from build123d import *

# Parameters (mm, degrees)
BOSS_EXTRUDE1_DEPTH = 400
SKETCH3_W           = 100
SKETCH3_H           = 300
CUT_EXTRUDE1_DEPTH  = 400
SKETCH4_W           = 60
SKETCH4_H           = 340
CUT_EXTRUDE2_DEPTH  = 400
SKETCH5_W           = 70
SKETCH5_H           = 340
CUT_EXTRUDE4_DEPTH  = 118
SKETCH6_R           = 5
CUT_EXTRUDE5_DEPTH  = 543
SKETCH7_R           = 5
CUT_EXTRUDE6_DEPTH  = 193
SKETCH8_R           = 10
CUT_EXTRUDE7_DEPTH  = 20
SKETCH9_W           = 100
SKETCH9_H           = 180
BOSS_EXTRUDE2_DEPTH = 20
SKETCH11_R          = 1
CUT_EXTRUDE8_DEPTH  = 26.5
SKETCH12_R          = 3.5
CUT_EXTRUDE9_DEPTH  = 35


with BuildPart() as part:
    # Sketch2 → Boss-Extrude1 (new body)
    with BuildSketch(Plane(origin=(0, 0, 0), x_dir=(1, 0, 0), z_dir=(0, 1, 0))):
        Polygon((0, 0), (0, 100), (20, 100), (20, 20), (180, 20), (180, 150), (200, 150), (200, 0), align=None)
    extrude(amount=-BOSS_EXTRUDE1_DEPTH)

    # Sketch3 → Cut-Extrude1 (cut)
    with BuildSketch(Plane.XY):
        with Locations((100, -200)):
            Rectangle(SKETCH3_W, SKETCH3_H)
    extrude(amount=-CUT_EXTRUDE1_DEPTH, mode=Mode.SUBTRACT)

    # Sketch4 → Cut-Extrude2 (cut)
    with BuildSketch(Plane.ZY):
        with Locations((-50, -200)):
            Rectangle(SKETCH4_W, SKETCH4_H)
    extrude(amount=-CUT_EXTRUDE2_DEPTH, mode=Mode.SUBTRACT)

    # Sketch5 → Cut-Extrude4 (cut)
    with BuildSketch(Plane(origin=(200, 0, 0), x_dir=(0, 0, -1), z_dir=(1, 0, 0))):
        with Locations((115, -200)):
            Rectangle(SKETCH5_W, SKETCH5_H)
    extrude(amount=-CUT_EXTRUDE4_DEPTH, mode=Mode.SUBTRACT)

    # Sketch6 → Cut-Extrude5 (cut)
    with BuildSketch(Plane(origin=(0, 0, 0), x_dir=(1, 0, 0), z_dir=(0, 1, 0))):
        with Locations(Location((190, 142, 0), (0, 0, 90))):
            Circle(SKETCH6_R)
        with Locations(Location((190, 129, 0), (0, 0, 90))):
            Circle(SKETCH6_R)
        with Locations(Location((190, 116, 0), (0, 0, 90))):
            Circle(SKETCH6_R)
        with Locations(Location((190, 103, 0), (0, 0, 90))):
            Circle(SKETCH6_R)
        with Locations(Location((190, 90, 0), (0, 0, 90))):
            Circle(SKETCH6_R)
    extrude(amount=-CUT_EXTRUDE5_DEPTH, mode=Mode.SUBTRACT)

    # Sketch7 → Cut-Extrude6 (cut)
    with BuildSketch(Plane.ZY):
        with Locations((-90, -80)):
            Circle(SKETCH7_R)
        with Locations((-90, -320)):
            Circle(SKETCH7_R)
    extrude(amount=-CUT_EXTRUDE6_DEPTH, mode=Mode.SUBTRACT)

    # Sketch8 → Cut-Extrude7 (cut)
    with BuildSketch(Plane.XY):
        with Locations((180, -60)):
            Circle(SKETCH8_R)
        with Locations((20, -60)):
            Circle(SKETCH8_R)
        with Locations((180, -340)):
            Circle(SKETCH8_R)
        with Locations((20, -340)):
            Circle(SKETCH8_R)
    extrude(amount=-CUT_EXTRUDE7_DEPTH, mode=Mode.SUBTRACT)

    # Sketch9 → Boss-Extrude2 (add)
    with BuildSketch(Plane.XY):
        with Locations((100, -200)):
            Rectangle(SKETCH9_W, SKETCH9_H)
    extrude(amount=-BOSS_EXTRUDE2_DEPTH)

    # Sketch11 → Cut-Extrude8 (cut, symmetric)
    with BuildSketch(Plane.XY):
        with Locations((75, -220)):
            Circle(SKETCH11_R)
        with Locations((123.17, -220)):
            Circle(SKETCH11_R)
    extrude(amount=CUT_EXTRUDE8_DEPTH, both=True, mode=Mode.SUBTRACT)

    # Sketch12 → Cut-Extrude9 (cut)
    with BuildSketch(Plane.XY):
        with Locations((190, -185)):
            Circle(SKETCH12_R)
    cut_extrude9 = extrude(amount=-CUT_EXTRUDE9_DEPTH, mode=Mode.SUBTRACT)

    # Mirror1: Cut-Extrude9 across plane
    add(cut_extrude9.mirror(Plane(origin=(100, 0, 0), x_dir=(0, 0, 1), z_dir=(1, 0, 0))), mode=Mode.SUBTRACT)


solid = part.part
Design review of the part built by this model. Coordinates are the model's own, in mm. A direction names the side the tool comes from. Coordinates: 2 decimals unless noted, no trailing zeros. Order: outer loops, then holes, each group sorted by start corner. A loop starts at its lowest first (then second) coordinate and runs counter-clockwise, first axis right, second up. Notation, with made-up numbers: M -27,41.25 L 19,41.25 A23 ccw 19,73.25 Z; hole C -19.75,7.25 d5. An arc over 180 degrees is marked long. Use a Markdown table: item, result.
(1) Add section B-B (z = -129). Give the boundary of the cut face in (x, y).
Worked answers:
| item | result |
|---|---|
| outline | M 180,-400 L 185,-400 L 185,-370 L 180,-370 Z; M 180,-30 L 185,-30 L 185,0 L 180,0 Z; M 195,-400 L 200,-400 L 200,-370 L 195,-370 Z; M 195,-30 L 200,-30 L 200,0 L 195,0 Z |
(2) Wall thickness on probe 1 along Y at (x, z) = (119.5, -14); probe 2 along Y at (x, z) = (180, -13); probe 3 along X at (y, z) = (-185, -3.75): over which ranges is each line inside the solid? List them lowest first.
Worked answers:
| item | result |
|---|---|
| probe 1 | y = -400 to -350, -290 to -110, -50 to 0 |
| probe 2 | y = -400 to -350, -330 to -70, -50 to 0 |
| probe 3 | x = 0 to 6.5, 13.5 to 186.5, 193.5 to 200 |
(3) Add section C-C (y = -195). Give the boundary of the cut face in (x, z), then the cut area to 3 significant figures.
Worked answers:
| item | result |
|---|---|
| outline | M 0,-100 L 20,-100 L 20,-80 L 0,-80 Z; M 0,-20 L 200,-20 L 200,0 L 0,0 Z |
| area | 4,400 mm2 |
(4) Add section A-A (y = -80). Give the boundary of the cut face in (x, z).
Worked answers:
| item | result |
|---|---|
| outline | M 0,-100 L 20,-100 L 20,-95 L 0,-95 Z; M 0,-85 L 20,-85 L 20,-80 L 0,-80 Z; M 0,-20 L 50,-20 L 50,0 L 0,0 Z; M 150,-20 L 200,-20 L 200,0 L 150,0 Z |
(5) For faces 4 (the cylindrical face through (18.698, -330.085, -9.86)), 5 (the flat face through (180, -15, -84)), 6 (the flat face through (150, -80, -10)), list the 3-axis set-ups (+Z, -Z, +X, -X, +Y, -Y) from which the entire face can be reached by the end or side of a thin tool; tool diameter is ignored.
Worked answers:
| item | result |
|---|---|
| face 4 | +Z |
| face 5 | -Z, +Y, -Y |
| face 6 | +Z, -Z |
(6) For P1, Ø2.5, axis at x = 123.17, y = -220, coming from the -Z side; P2, Ø6.5, axis at x = 10, y = -185, coming from the -Z side; P3, Ø12, axis at x = 20, y = -340, coming from the +Z side, all flat-tipped, find the tip position at first contact; note any pin that passes through.
Worked answers:
| item | result |
|---|---|
| P1 | stops at z = -20 |
| P2 | stops at z = -100 |
| P3 | stops at z = -80 |
(7) Add section D-D (x = 108). Give the boundary of the cut face in (y, z), then the cut area to 3 significant figures.
Worked answers:
| item | result |
|---|---|
| outline | M -400,-20 L -350,-20 L -350,0 L -400,0 Z; M -290,-20 L -110,-20 L -110,0 L -290,0 Z; M -50,-20 L 0,-20 L 0,0 L -50,0 Z |
| area | 5,600 mm2 |
(8) Draft analysis for pull direction Z (two halves, no side actions). For faces 1 (the flat face through (101, -197, 0)), 2 (the flat face through (200, -199.1, -19.8)), 3 (the cylindrical face through (185.043, -14.79, -141.349)), state which applies: released by +Z, released by -Z, zero draft, split by the parting line, or undercut.
Worked answers:
| item | result |
|---|---|
| face 1 | released by +Z |
| face 2 | zero draft |
| face 3 | undercut |
